Source: CAD feature listing. Evaluate the final solid. Frame: model axes, mm. A direction names the side the tool comes from. Round coordinates to 2 decimals unless told otherwise and drop trailing zeros. Write each loop counter-clockwise with the first axis right and the second up, starting at its lowest first coordinate (ties: lowest second). Pieces come first, ordered by that corner, then holes.
Autodesk Inventor part; units mm, degrees
ref_plane "YZ Plane" through (0, 0, 0) normal (1, 0, 0) x (0, 1, 0)
ref_plane "XZ Plane" through (0, 0, 0) normal (0, 1, 0) x (-1, 0, 0)
ref_plane "XY Plane" through (0, 0, 0) normal (0, 0, 1) x (1, 0, 0)
sketch "Sketch1" plane through (0, 0, 0) normal (1, 0, 0) x (0, 1, 0)
  line L0 (0, 0) -> (50.8, 0)
  line L1 (50.8, 0) -> (50.8, -76.2)
  line L2 (50.8, -76.2) -> (0, -76.2)
  line L3 (0, -76.2) -> (0, 0)
  dimension "d0" = 76.2
  dimension "d1" = 50.8
extrude "Extrusion1" add sketch "Sketch1" along normal blind 50.8
shell "Shell1" thickness 3.175 removed faces 2 at (0, 33.8667, -50.8) at (50.8, 33.8667, -50.8)
fillet "Fillet1" radius 3.175 8 edges at (25.4, 3.175, -3.175) (25.4, 3.175, -73.025) (25.4, 47.625, -3.175) (25.4, 47.625, -73.025) (25.4, 50.8, 0) (25.4, 0, 0) (25.4, 50.8, -76.2) (25.4, 0, -76.2)
sketch "Sketch2" plane through (0, 0, -73.025) normal (0, -1, 0) x (1, 0, 0)
  circle A0 centre (12.5, 11.825) radius 3.175
  circle A1 centre (12.5, 58.025) radius 3.175
  circle A2 centre (38.3, 11.825) radius 3.175
  circle A3 centre (38.3, 58.025) radius 3.175
  line L0 (12.5, 11.825) -> (38.3, 11.825) construction
  line L1 (38.3, 11.825) -> (38.3, 58.025) construction
  line L2 (38.3, 58.025) -> (12.5, 58.025) construction
  line L3 (12.5, 58.025) -> (12.5, 11.825) construction
  line L4 (0, 73.025) -> (50.8, 73.025) construction
  line L5 (50.8, 73.025) -> (50.8, -3.175) construction
  line L6 (50.8, -3.175) -> (0, -3.175) construction
  line L7 (0, -3.175) -> (0, 73.025) construction
  point P0 (25.4, 58.025)
  point P1 (25.4, 73.025)
  point P2 (12.5, 34.925)
  point P3 (0, 34.925)
  dimension "d6" = 6.35
  dimension "d7" = 50.8
  dimension "d8" = 76.2
  dimension "d10" = 12.5
  dimension "d11" = 15
extrude "Extrusion2" cut sketch "Sketch2" against normal up to surface (3.175 mm away)
sketch "Sketch3" plane through (0, 50.8, -3.175) normal (0, 1, 0) x (1, 0, 0)
  line L0 (0, -3.175) -> (50.8, -3.175) construction
  line L1 (50.8, -3.175) -> (50.8, 73.025) construction
  line L2 (50.8, 73.025) -> (0, 73.025) construction
  line L3 (0, 73.025) -> (0, -3.175) construction
  line L4 (47.625, 73.025) -> (47.625, -3.175) construction
  line L5 (3.175, -3.175) -> (3.175, 73.025) construction
  line L6 (47.625, 34.925) -> (50.8, 34.925) construction
  line L7 (3.175, 34.925) -> (0, 34.925) construction
  line L8 (37.9, 53.025) -> (12.9, 53.025) construction
  line L9 (12.9, 53.025) -> (12.9, 16.825) construction
  line L10 (12.9, 16.825) -> (37.9, 16.825) construction
  line L11 (37.9, 16.825) -> (37.9, 53.025) construction
  circle A0 centre (25.4, 53.025) radius 3.175
  circle A1 centre (12.9, 16.825) radius 3.175
  circle A2 centre (37.9, 16.825) radius 3.175
  line L12 (25.4, 16.825) -> (25.4, -3.175) construction
  line L13 (25.4, 53.025) -> (25.4, 73.025) construction
  dimension "d14" = 3.175
  dimension "d15" = 76.2
  dimension "d16" = 50.8
  dimension "d17" = 6.35
  dimension "d19" = 25
  dimension "d20" = 20
extrude "Extrusion3" cut sketch "Sketch3" against normal up to surface (3.175 mm away)
properties part number "3x2_Bar" material "Steel, Mild"
1) Reachability of faces 1 (the face through (40.007, 1.565, -58.523)), 2 (the face through (27.107, 49.235, -58.877)), 3 (the face through (25.04, 46.67, -4.08)) from +Z, -Z, +X, -X, +Y, -Y: full face, straight path, thin tool, end or side. Return the list, or none.
Taken from the geometry:
face 1: -Y
face 2: +Y
face 3: +X, -X
2) Pull-direction query (X, two-part tool) for faces 4 (the face through (50.8, 3, -35)), 5 (the face through (25, 25, -3.175)), 6 (the face through (15.83, 49.23, -18.78)); classes: released by +X, released by -X, zero draft, split by the parting line, or undercut.
Taken from the geometry:
face 4: released by +X
face 5: zero draft
face 6: undercut
3) Section query C-C on x = 6. Return the cut outline in (y, z) (3 decimals).
Taken from the geometry:
outline: (0, -73.025) arc R3.175 ccw to (3.175, -76.2) - (47.625, -76.2) arc R3.175 ccw to (50.8, -73.025) - (50.8, -3.175) arc R3.175 ccw to (47.625, 0) - (3.175, 0) arc R3.175 ccw to (0, -3.175) - close; hole (3.175, -69.85) arc R3.175 ccw to (6.35, -73.025) - (44.45, -73.025) arc R3.175 ccw to (47.625, -69.85) - (47.625, -6.35) arc R3.175 ccw to (44.45, -3.175) - (6.35, -3.175) arc R3.175 ccw to (3.175, -6.35) - close
4) Material intervals for line 1 (X direction, y = 48.7, z = -20) (3 decimals); line 2 (Y direction, x = 28.5, z = -43) (3 decimals); line 3 (Z direction, x = 19, y = 29) (3 decimals), sorted ascending.
Taken from the geometry:
line 1: x = 0 to 9.725, 16.075 to 34.725, 41.075 to 50.8
line 2: y = 0 to 3.175, 47.625 to 50.8
line 3: z = -76.2 to -73.025, -3.175 to 0
5) Section query B-B on z = -49. Return the cut outline in (x, y) (3 decimals), then the cut area to 3 significant figures.
Taken from the geometry:
outline: (0, 0) - (50.8, 0) - (50.8, 3.175) - (0, 3.175) - close; (0, 47.625) - (50.8, 47.625) - (50.8, 50.8) - (0, 50.8) - close
area: 323 mm2
6) Section query D-D on y = 11. Return the cut outline in (x, z) (3 decimals).
Taken from the geometry:
outline: (0, -76.2) - (50.8, -76.2) - (50.8, -73.025) - (0, -73.025) - close; (0, -3.175) - (50.8, -3.175) - (50.8, 0) - (0, 0) - close
7) Section query A-A on z = -61.2. Return the cut outline in (x, y) (3 decimals).
Taken from the geometry:
outline: (0, 0) - (9.325, 0) - (9.325, 3.175) - (0, 3.175) - close; (0, 47.625) - (50.8, 47.625) - (50.8, 50.8) - (0, 50.8) - close; (15.675, 0) - (35.125, 0) - (35.125, 3.175) - (15.675, 3.175) - close; (41.475, 0) - (50.8, 0) - (50.8, 3.175) - (41.475, 3.175) - close
8) Contact query for flat-ended pins moving along their axis: P1, Ø5, axis at x = 12.9, z = -20, coming from the +Y side (3 decimals); P2, Ø4, axis at x = 38.3, z = -61.2, coming from the -Y side (3 decimals). Output: stop coordinate, or through.
Taken from the geometry:
P1: stops at y = 3.175
P2: stops at y = 47.625
